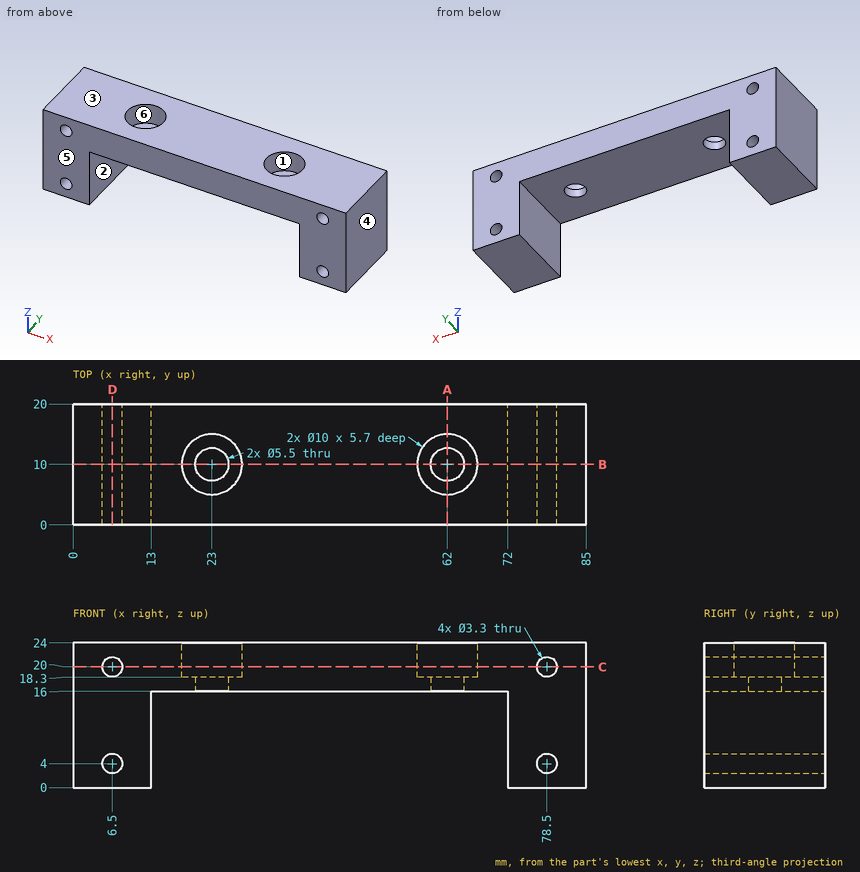
Job drawing, mm, ordinate dimensions from the low corner. One solid piece. A direction names the side the tool comes from. Round coordinates to 2 decimals unless told otherwise and drop trailing zeros. Loops run counter-clockwise (first coordinate to the right, second up) from the corner with the lowest first, then second, coordinate; pieces in that order, holes last. Notation, with made-up numbers: M -17,-27.75 L -6,-27.75 A21 ccw -6,-9.75 Z; hole C 80,74.25 d8. An arc over 180 degrees is marked long. Answer as CSV lines item,"result".
1. Wall check: probe 1 along Z at (x, y) = (78.5, 11.25); probe 2 along X at (y, z) = (1.75, 20.25); probe 3 along Y at (x, z) = (23, 21.15). Give the ranges that are in metal, low to high. Write a range as [from, to].
Resolved:
probe 1,"z = [0, 2.35], [5.65, 18.35], [21.65, 24]"
probe 2,"x = [0, 4.87], [8.13, 76.87], [80.13, 85]"
probe 3,"y = [0, 5], [15, 20]"
2. Flat gauge pins, fed straight in: P1, Ø12, axis at y = 12.5, z = 7, coming from the -X side; P2, Ø3, axis at x = 61, y = 11.5, coming from the +Z side; P3, Ø7, axis at x = 62, y = 10, coming from the -Z side. Where does each tip first touch, or does it go through?
Resolved:
P1,"stops at x = 0"
P2,"stops at z = 18.3"
P3,"stops at z = 16"
3. Cut at B-B on y = 10. Write the cut outline in (x, z), then the cut area to 3 significant figures.
Resolved:
outline,"M 0,0 L 13,0 L 13,16 L 20.25,16 L 20.25,18.3 L 18,18.3 L 18,24 L 0,24 Z; M 25.75,16 L 59.25,16 L 59.25,18.3 L 57,18.3 L 57,24 L 28,24 L 28,18.3 L 25.75,18.3 Z; M 64.75,16 L 72,16 L 72,0 L 85,0 L 85,24 L 67,24 L 67,18.3 L 64.75,18.3 Z; hole C 6.5,4 d3.3; hole C 6.5,20 d3.3; hole C 78.5,4 d3.3; hole C 78.5,20 d3.3"
area,"922 mm²"
4. Cut at C-C on z = 20. Write the cut outline in (x, y).
Resolved:
outline,"M 0,0 L 4.85,0 L 4.85,20 L 0,20 Z; M 8.15,0 L 76.85,0 L 76.85,20 L 8.15,20 Z; M 80.15,0 L 85,0 L 85,20 L 80.15,20 Z; hole C 23,10 d10; hole C 62,10 d10"
5. Cut at A-A on x = 62. Write the cut outline in (y, z), then the cut area to 4 significant figures.
Resolved:
outline,"M 0,16 L 7.25,16 L 7.25,18.3 L 5,18.3 L 5,24 L 0,24 Z; M 12.75,16 L 20,16 L 20,24 L 15,24 L 15,18.3 L 12.75,18.3 Z"
area,"90.35 mm²"
6. 3-axis set-ups, long thin cutter, end or side, ignore diameter. For the marked faces 1, 2 and 3: which of +Z, -Z, +X, -X, +Y, -Y reach the whole face in a straight line?
Resolved:
face 1,"+Z"
face 2,"-Z, +Y, -Y"
face 3,"+Z, +X, -X, +Y, -Y"
7. Two-plate mould, pull along X, no slides. Class the marked faces 4, 5 and 6: released by +X, released by -X, zero draft, split by the parting line, or undercut.
Resolved:
face 4,"released by +X"
face 5,"zero draft"
face 6,"undercut"
8. Cut at D-D on x = 6.5. Write the cut outline in (y, z), then the cut area to 3 significant figures.
Resolved:
outline,"M 0,0 L 20,0 L 20,2.35 L 0,2.35 Z; M 0,5.65 L 20,5.65 L 20,18.35 L 0,18.35 Z; M 0,21.65 L 20,21.65 L 20,24 L 0,24 Z"
area,"348 mm²"
